from build123d import *

# Parameters (mm, degrees)
F0_W         = 76.2
F0_H         = 38.1
F1_DEPTH     = 25.4
F2_R         = 12.7
F3_R         = 5.08
F4_R         = 5.08
F5_DEPTH     = 25.4
F6_R         = 5.08
F7_DEPTH     = 25.4
F8_W         = 66.04
F8_H         = 25.4
F9_DEPTH     = 19.05
F10_W        = 66.04
F10_H        = 3.175
F11_DEPTH    = 12.7
F12_T1_DEPTH = 66.04
F12_T6_DEPTH = 66.04


# Not quite as in the source:
# - a fillet or chamfer that OpenCascade refuses, or shapes differently, is made with other operations: its cross-section is extruded or revolved along the edge and cut away or added


with BuildPart() as f1:
    # F0 (on Top) → F1 (new body)
    with BuildSketch(Plane.XY):
        with Locations((-1.7044725776, 2.5065781057)):
            Rectangle(F0_W, F0_H)
    extrude(amount=F1_DEPTH)

    # F2
    f2_edges = [f1.edges().sort_by_distance(p)[0] for p in [
        (-39.804473, 21.556578, 12.7),
        (36.395527, 21.556578, 12.7),
    ]]
    fillet(f2_edges, radius=F2_R)

    # F3
    f3_edges = [f1.edges().sort_by_distance(p)[0] for p in [
        (-39.804473, -16.543422, 12.7),
        (36.395527, -16.543422, 12.7),
    ]]
    fillet(f3_edges, radius=F3_R)

    # F4 (on face) → F5 (join)
    with BuildSketch(Plane(origin=(-39.8044725776, 0, 0), x_dir=(0, -1, 0), z_dir=(-1, 0, 0))):
        with Locations((0, 12.7)):
            Circle(F4_R)
    extrude(amount=F5_DEPTH)

    # F6 (on face) → F7 (join)
    with BuildSketch(Plane.YZ.offset(36.3955274224)):
        with Locations((0, 13.3897410706)):
            Circle(F6_R)
    extrude(amount=F7_DEPTH)

    # F8 (on face) → F9 (cut)
    with BuildSketch(Plane.XY.offset(25.4)):
        with Locations((-1.7044725776, 1.2365781057)):
            Rectangle(F8_W, F8_H)
    extrude(amount=-F9_DEPTH, mode=Mode.SUBTRACT)

    # F10 (on face) → F11 (join)
    with BuildSketch(Plane.XY.offset(6.35)):
        with Locations((-1.7044725776, 9.1740781057)):
            Rectangle(F10_W, F10_H)
        with Locations((-1.7044725776, 2.8240781057)):
            Rectangle(F10_W, F10_H)
        with Locations((-1.7044725776, -3.5259218943)):
            Rectangle(F10_W, F10_H)
        with Locations((-1.7044725776, -9.8759218943)):
            Rectangle(F10_W, F10_H)
    extrude(amount=F11_DEPTH)

    # F12: chamfer of 5.08 on 4 edges, made by hand

    # F12_s2 → F12_t1 (cut)
    with BuildSketch(Plane.YZ.offset(-34.7244725776)):
        Polygon((5.6815781057, 19.05), (10.7615781057, 13.97), (10.7615781057, 19.05), align=None)
        Polygon((-0.6684218943, 19.05), (4.4115781057, 13.97), (4.4115781057, 19.05), align=None)
        Polygon((-7.0184218943, 19.05), (-1.9384218943, 13.97), (-1.9384218943, 19.05), align=None)
    extrude(amount=F12_T1_DEPTH, mode=Mode.SUBTRACT)


with BuildPart() as f12_tool4:
    # F12_s5 → F12_t6 (new body)
    with BuildSketch(Plane.YZ.offset(31.3155274224)):
        Polygon((-13.3684218943, 19.05), (-8.2884218943, 13.97), (-8.2884218943, 19.05), align=None)
    extrude(amount=-F12_T6_DEPTH)

    split(bisect_by=Plane.XZ.offset(11.4634218943), keep=Keep.BOTTOM)


with BuildPart() as f1_1:
    add(f1.part)

    # F12_t3: cut F12_tool4
    add(f12_tool4.part, mode=Mode.SUBTRACT)


solid = f1_1.part
The listing builds one solid part. Answer for the finished solid, in the listing's coordinates (mm). A direction names the side the tool comes from. Round coordinates to 2 decimals unless told otherwise and drop trailing zeros. Loops run counter-clockwise (first coordinate to the right, second up) from the corner with the lowest first, then second, coordinate; pieces in that order, holes last. Notation, with made-up numbers: M -1.5,29.25 L 15.5,29.25 A6 ccw 15.5,35.25 Z; hole C -14,-30.75 d6. An arc over 180 degrees is marked long. Return JSON: item names as keys, results as strings.
Q1. Each of these flat-tipped pins is pushed along its axis until it touches: pin 1 Ø2 at (x, y) = (-52, -3) entering from +Z; pin 2 Ø1.6 at (x, y) = (-8, 5.5) entering from +Z; pin 3 Ø8 at (y, z) = (9.5, 10) entering from +X. Where does it stop, or does it pass through?
Results list:
{"pin 1": "stops at z = 17.37", "pin 2": "stops at z = 6.35", "pin 3": "stops at x = 36.4"}
Q2. Find section B-B, the plane y = 0. Determine the outline of the cut face in (x, z), plus the area to 3 significant figures.
Results list:
{"outline": "M -65.2,7.62 L -39.8,7.62 L -39.8,0 L 36.4,0 L 36.4,8.31 L 61.8,8.31 L 61.8,18.47 L 36.4,18.47 L 36.4,25.4 L 31.32,25.4 L 31.32,6.35 L -34.72,6.35 L -34.72,25.4 L -39.8,25.4 L -39.8,17.78 L -65.2,17.78 Z", "area": "1,190 mm2"}
Q3. Find section C-C, the plane x = -8.5. Determine the outline of the cut face in (y, z) (3 decimals).
Results list:
{"outline": "M -16.543,0 L 21.557,0 L 21.557,25.4 L 13.937,25.4 L 13.937,6.35 L 10.762,6.35 L 10.762,13.97 L 7.587,17.145 L 7.587,6.35 L 4.412,6.35 L 4.412,13.97 L 1.237,17.145 L 1.237,6.35 L -1.938,6.35 L -1.938,13.97 L -5.113,17.145 L -5.113,6.35 L -8.288,6.35 L -8.288,13.97 L -11.463,17.145 L -11.463,25.4 L -16.543,25.4 Z"}
Q4. The mould has two halves that part along X. Classify faces 1 (the face through (61.796, 0, 13)), 2 (the face through (-39.804, -6, 13)), 3 (the face through (-2, 3, 0)), 4 (the face through (-2.17, -3.55, 15.58)): released by +X, released by -X, zero draft, split by the parting line, or undercut.
Results list:
{"face 1": "released by +X", "face 2": "released by -X", "face 3": "zero draft", "face 4": "undercut"}
Q5. Which of the six approach directions +Z, -Z, +X, -X, +Y, -Y give full straight-line access (tool end or side, diameter ignored) to faces 5 (the face through (-2, 21.557, 13)), 6 (the face through (-52.327, 0.661, 17.737)), 7 (the face through (-2, -7, 6.35))?
Results list:
{"face 5": "+Z, -Z, +X, -X, +Y", "face 6": "-X", "face 7": "+Z"}
Q6. Find section A-A, the plane z = 23.25. Determine the outline of the cut face in (x, y), plus the area to 3 significant figures.
Results list:
{"outline": "M -39.8,-11.46 A5.08 ccw -34.72,-16.54 L 31.32,-16.54 A5.08 ccw 36.4,-11.46 L 36.4,8.86 A12.7 ccw 23.7,21.56 L -27.1,21.56 A12.7 ccw -39.8,8.86 Z; hole M -34.72,-11.46 L 31.32,-11.46 L 31.32,13.94 L -34.72,13.94 Z", "area": "1,150 mm2"}
Q7. Find the intervals of material crossed by line 1 along Y through (x, z) = (2.5, 18); line 2 along X through (y, z) = (-0.5, 20); line 3 along Y through (x, z) = (-32, 7), in increasing order. Write a range as from..to.
Results list:
{"line 1": "y = -16.54..-11.46, 13.94..21.56", "line 2": "x = -39.8..-34.72, 31.32..36.4", "line 3": "y = -16.54..-8.29, -5.11..-1.94, 1.24..4.41, 7.59..10.76, 13.94..20.58"}
Q8. Find section D-D, the plane z = 4. Determine the outline of the cut face in (x, y), plus the area to 3 significant figures.
Results list:
{"outline": "M -39.8,-11.46 A5.08 ccw -34.72,-16.54 L 31.32,-16.54 A5.08 ccw 36.4,-11.46 L 36.4,8.86 A12.7 ccw 23.7,21.56 L -27.1,21.56 A12.7 ccw -39.8,8.86 Z", "area": "2,820 mm2"}
